Check sheet for the drawn part. Datum: minimum x, y, z corner. Units: mm. Coordinates: 2 decimals unless noted, no trailing zeros. Write each loop counter-clockwise with the first axis right and the second up, starting at its lowest first coordinate (ties: lowest second). Pieces come first, ordered by that corner, then holes. Notation, with made-up numbers: M -22.5,30.5 L 9.5,30.5 A16 cw 9.5,48.5 Z; hole C -19.5,16.5 d4. An arc over 180 degrees is marked long. Answer in a Markdown table with one row per item.
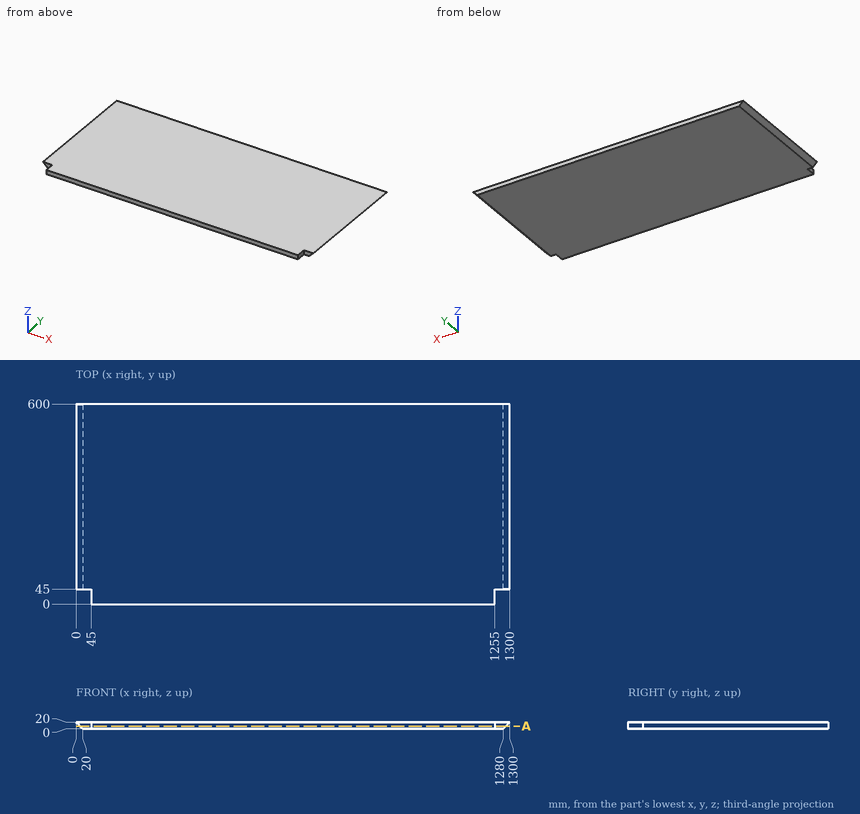
1) Sectioned sample at A-A (z = 8.5). Record the cut outline in (x, y).
Response values:
| item | result |
|---|---|
| outline | M 11.5,45 L 45,45 L 45,0 L 1255,0 L 1255,45 L 1288.5,45 L 1288.5,600 L 11.5,600 Z |
2) Thickness scan on L1, parallel to X at y = 122.5, z = 1.75; L2, parallel to X at y = 186, z = 12. Record the ranges inside material, lowest first. Write a range as [from, to].
Response values:
| item | result |
|---|---|
| L1 | x = [18.25, 1281.75] |
| L2 | x = [8, 1292] |
3) Depth check by flat-ended pin: pin 1 (3 mm diameter, centred on y = 135, z = 3.5, fed in from +X); pin 2 (10 mm diameter, centred on y = 31.5, z = 15, fed in from +X); pin 3 (2 mm diameter, centred on y = 170.5, z = 3, fed in from +X). Enter the tip coordinate at first touch or a pass-through.
Response values:
| item | result |
|---|---|
| pin 1 | stops at x = 1285 |
| pin 2 | stops at x = 1255 |
| pin 3 | stops at x = 1284 |
